The model under review builds one solid part; all positions refer to its coordinate system, in mm. Round coordinates to 2 decimals unless told otherwise and drop trailing zeros. Order: outer loops, then holes, each group sorted by start corner. A loop starts at its lowest first (then second) coordinate and runs counter-clockwise, first axis right, second up. Notation, with made-up numbers: (-40, 63.25) -> (-30, 63.25) arc R24 ccw to (-30, 102.25) -> close; hole circle Ø1 at (16, 63). An arc over 180 degrees is marked (long way). Return JSON: item names as keys, results as strings. Group by question number.
from build123d import *

# Parameters (mm, degrees)
SKETCH1_W           = 3
SKETCH1_H           = 10
SKETCH1_W_2         = 10
SKETCH1_H_2         = 3
BOSS_EXTRUDE1_DEPTH = 3
FILLET1_R           = 3


with BuildPart() as part:
    # Sketch1 → Boss-Extrude1 (new body)
    with BuildSketch(Plane(origin=(0, 0, 0), x_dir=(1, 0, 0), z_dir=(0, 1, 0))):
        Polygon((0, 29), (0, 0), (100, 0), (110, 0), (110, 29), (110, 39), (110, 42), (107, 42), (107, 40.5), (104, 40.5), (104, 42), (95, 42), (95, 45), (104, 45), (104, 46.5), (107, 46.5), (107, 45), (110, 45), (110, 48), (110, 58), (110, 83.95), (69.5, 83.95), (59.5, 83.95), (56.5, 83.95), (56.5, 80.95), (58, 80.95), (58, 77.95), (56.5, 77.95), (56.5, 68.95), (53.5, 68.95), (53.5, 77.95), (52, 77.95), (52, 80.95), (53.5, 80.95), (53.5, 83.95), (50.5, 83.95), (40.5, 83.95), (0, 83.95), (0, 58), (0, 48), (0, 45), (3, 45), (3, 46.5), (6, 46.5), (6, 45), (15, 45), (15, 42), (6, 42), (6, 40.5), (3, 40.5), (3, 42), (0, 42), (0, 39), align=None)
        with Locations((-1.5, 53)):
            Rectangle(SKETCH1_W, SKETCH1_H)
        with Locations((-1.5, 34)):
            Rectangle(SKETCH1_W, SKETCH1_H)
        with Locations((45.5, 85.45)):
            Rectangle(SKETCH1_W_2, SKETCH1_H_2)
        with Locations((64.5, 85.45)):
            Rectangle(SKETCH1_W_2, SKETCH1_H_2)
        with Locations((111.5, 53)):
            Rectangle(SKETCH1_W, SKETCH1_H)
        with Locations((111.5, 34)):
            Rectangle(SKETCH1_W, SKETCH1_H)
    extrude(amount=BOSS_EXTRUDE1_DEPTH)

    # Fillet1
    fillet1_edges = [part.edges().sort_by_distance(p)[0] for p in [
        (110, 1.5, -83.95),
        (110, 1.5, 0),
        (0, 1.5, 0),
        (0, 1.5, -83.95),
    ]]
    fillet(fillet1_edges, radius=FILLET1_R)


solid = part.part
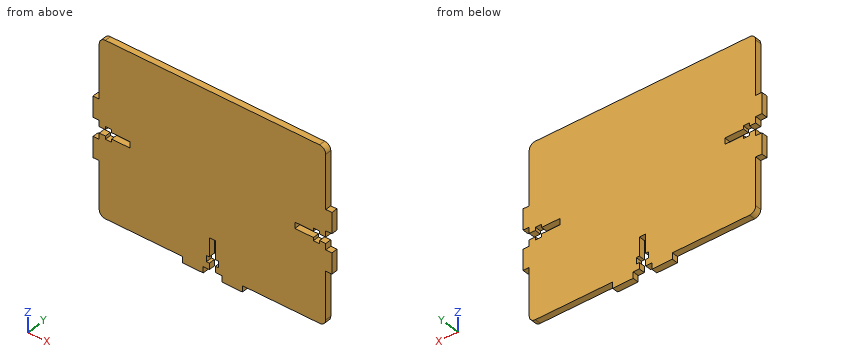
Item 1: Consider section C-C on x = 74.5. State the section outline as (y, z) points.
Item 2: Consider section D-D on z = -22. State the section outline as (x, y) points.
Item 3: Consider section B-B on x = 12. State the section outline as (y, z) points.
Item 4: Wall thickness on line 1 along Z through (x, y) = (96, 1.7); line 2 along X through (y, z) = (1.4, -20); line 3 along Z through (x, y) = (20, 0.35): over which ranges is each line inside the solid? List them lowest first.
Item 5: Consider section A-A on z = -76.5. State the section outline as (x, y) points.
Item 6: Insertion check: pin 1 Ø1.5 at (x, y) = (111, 1) entering from -Z; pin 2 Ø1.5 at (y, z) = (1, -18) entering from +X; pin 3 Ø0.9 at (y, z) = (2, -40.5) entering from -X. Each pin has a flat end and moves straight along its axis. Give the tip position at first contact, or say it passes through.
Values:
{
 "1": {"outline": "(0, -83.95) -> (3, -83.95) -> (3, 0) -> (0, 0) -> close"},
 "2": {"outline": "(0, 0) -> (110, 0) -> (110, 3) -> (0, 3) -> close"},
 "3": {"outline": "(0, -83.95) -> (3, -83.95) -> (3, -45) -> (0, -45) -> close; (0, -42) -> (3, -42) -> (3, 0) -> (0, 0) -> close"},
 "4": {"line 1": "-83.95 to -45, -42 to 0", "line 2": "0 to 110", "line 3": "-83.95 to 0"},
 "5": {"outline": "(0, 0) -> (53.5, 0) -> (53.5, 3) -> (0, 3) -> close; (56.5, 0) -> (110, 0) -> (110, 3) -> (56.5, 3) -> close"},
 "6": {"pin 1": "z = -58", "pin 2": "x = 110", "pin 3": "x = 0"}
}
